Check sheet for the modelled part. Datum: model origin and axes. Units: mm. Face numbers are marked on the shaded views. A direction names the side the tool comes from. Round coordinates to 2 decimals unless told otherwise and drop trailing zeros. Write each loop counter-clockwise with the first axis right and the second up, starting at its lowest first coordinate (ties: lowest second). Pieces come first, ordered by that corner, then holes.
Item 1: Cross-section at A-A on y = 5. Enter the section's corners in (x, z), plus the area to 3 significant figures.
Item 2: Material ranges on line 1 (Y direction, x = -2.5, z = 0); line 2 (X direction, y = 0.75, z = 0); line 3 (X direction, y = 6.25, z = 4.75), recorded low to high.
Item 3: Tool access check on the marked faces 1, 2 and 3. Record the directions out of +Z, -Z, +X, -X, +Y, -Y that give a thin tool (end or side, any length) a straight path to the whole face; none if there is none.
Item 4: Release check for a two-part mould opening along X. For the marked faces 4, 5, 6 and 7 record: +X half, -X half, draft (parallel to the pull), parting line (faces both ways), or undercut.
Item 5: Cross-section at B-B on z = 0. Enter the section's corners in (x, y), plus the area to 3 significant figures.
Item 6: Cross-section at D-D on x = -8.5. Enter the section's corners in (y, z), plus the area to 3 significant figures.
Item 7: Cross-section at C-C on x = -2.75. Enter the section's corners in (y, z), plus the area to 3 significant figures.
Item 8: Go/stop test with flat-tipped pins: pin 1 Ø1 at (x, y) = (-7, 5) entering from -Z; pin 2 Ø3 at (x, z) = (-3, 4.5) entering from -Y. Record where each tip stops, or that it passes through.
from build123d import *

# Parameters (mm, degrees)
SKETCH2_W               = 8
SKETCH2_H               = 10
BOSS_EXTRUDE1_DEPTH     = 8
SKETCH4_W               = 19
SKETCH4_H               = 10
BOSS_EXTRUDE2_DEPTH     = 2
SKETCH6_W               = 19
SKETCH6_H               = 4
BOSS_EXTRUDE3_DEPTH     = 1
SKETCH7_W               = 1
SKETCH7_H               = 10
BOSS_EXTRUDE4_DEPTH     = 2
CUT_EXTRUDE1_REACH      = 24.293
SKETCH3_R               = 2.5
CUT_EXTRUDE2_REACH      = 21
CUT_EXTRUDE2_END_RADIUS = 2.5
SKETCH8_R               = 1
FILLET3_R               = 4
SKETCH9_W               = 10
SKETCH9_H               = 10
CUT_EXTRUDE3_DEPTH      = 0.5


with BuildPart() as part:
    # Sketch2 → Boss-Extrude1 (new body)
    with BuildSketch(Plane(origin=(0, 0, 0), x_dir=(1, 0, 0), z_dir=(0, 1, 0))):
        Rectangle(SKETCH2_W, SKETCH2_H)
    extrude(amount=BOSS_EXTRUDE1_DEPTH)

    # Sketch4 → Boss-Extrude2 (add)
    with BuildSketch(Plane(origin=(0, 8, 0), x_dir=(1, 0, 0), z_dir=(0, 1, 0))):
        with Locations((-5.5, 0)):
            Rectangle(SKETCH4_W, SKETCH4_H)
    extrude(amount=BOSS_EXTRUDE2_DEPTH)

    # Sketch6 → Boss-Extrude3 (add)
    with BuildSketch(Plane.XY.offset(5)):
        with Locations((-5.5, 8)):
            Rectangle(SKETCH6_W, SKETCH6_H)
    boss_extrude3 = extrude(amount=BOSS_EXTRUDE3_DEPTH)

    # Mirror1: Boss-Extrude3 across plane
    add(boss_extrude3.mirror(Plane.XY))

    # Sketch7 → Boss-Extrude4 (add)
    with BuildSketch(Plane.XZ.offset(-8)):
        with Locations((-14.5, 0)):
            Rectangle(SKETCH7_W, SKETCH7_H)
    extrude(amount=BOSS_EXTRUDE4_DEPTH)

    # Sketch3 → Cut-Extrude1 (cut, up to next)
    with BuildSketch(Plane(origin=(4, 0, 0), x_dir=(0, 0, -1), z_dir=(1, 0, 0)), mode=Mode.PRIVATE) as cut_extrude1_sk1:
        with Locations((0, 5)):
            Circle(SKETCH3_R)
    cut_extrude1_tool1 = extrude(cut_extrude1_sk1.sketch, amount=-CUT_EXTRUDE1_REACH, mode=Mode.PRIVATE) & part.part
    add(cut_extrude1_tool1.solids().sort_by_distance((4, 5, 0))[0], mode=Mode.SUBTRACT)

    # Cut-Extrude2: up to this cylinder (the profile starts outside it)
    cut_extrude2_end = Plane(origin=(0, 5, 0), z_dir=(1, 0, 0)) * Cylinder(CUT_EXTRUDE2_END_RADIUS, 48, mode=Mode.PRIVATE)
    # Sketch8 → Cut-Extrude2 (cut, up to the surface)
    with BuildSketch(Plane.XZ, mode=Mode.PRIVATE) as cut_extrude2_sk1:
        with Locations(Location((0, 0, 0), (0, 0, 270))):
            Circle(SKETCH8_R)
    cut_extrude2_tool1 = extrude(cut_extrude2_sk1.sketch, amount=-CUT_EXTRUDE2_REACH, mode=Mode.PRIVATE) - cut_extrude2_end
    add(cut_extrude2_tool1.solids().sort_by_distance((0, 0, 0))[0], mode=Mode.SUBTRACT)

    # Fillet3
    fillet3_edges = [part.edges().sort_by_distance(p)[0] for p in [
        (0, 0, 5),
        (0, 0, -5),
    ]]
    fillet(fillet3_edges, radius=FILLET3_R - 0.0001)  # a hair under: the kernel refuses the full size

    # Sketch9 → Cut-Extrude3 (cut)
    with BuildSketch(Plane(origin=(0, 10, 0), x_dir=(1, 0, 0), z_dir=(0, 1, 0))):
        with Locations((-9, 0)):
            Rectangle(SKETCH9_W, SKETCH9_H)
    extrude(amount=-CUT_EXTRUDE3_DEPTH, mode=Mode.SUBTRACT)


solid = part.part
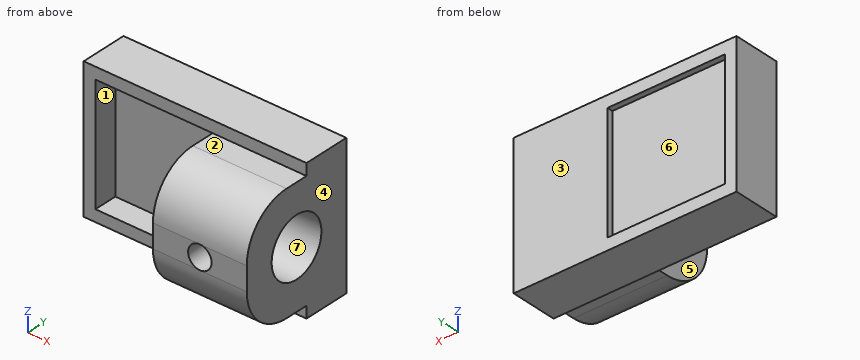
Response values:
1. outline: (-4, -5) - (4, -5) - (4, -2.5) - (-4, -2.5) - close; (-4, 2.5) - (4, 2.5) - (4, 5) - (-4, 5) - close
1. area: 40.0 mm2
2. line 1: y = 0 to 2.5, 7.5 to 10
2. line 2: x = -4 to -1, 1 to 4
2. line 3: x = -15 to -14, -4 to 4
3. face 1: -Y
3. face 2: +Z, +X, -X, -Y
3. face 3: +Z, -Z, +X, -X, +Y
4. face 4: +X half
4. face 5: undercut
4. face 6: undercut
4. face 7: draft
5. outline: (-15, 6) - (-14, 6) - (-14, 8) - (-4, 8) - (-4, 7.5) - (4, 7.5) - (4, 10) - (-4, 10) - (-4, 9.5) - (-14, 9.5) - (-14, 10) - (-15, 10) - close; (-4, 0) - (-1, 0) - (-1, 2.5) - (-4, 2.5) - close; (1, 0) - (4, 0) - (4, 2.5) - (1, 2.5) - close
5. area: 54.0 mm2
6. outline: (6, -6) - (10, -6) - (10, -5) - (9.5, -5) - (9.5, 5) - (10, 5) - (10, 6) - (6, 6) - (6, 5) - (8, 5) - (8, -5) - (6, -5) - close
6. area: 23.0 mm2
7. outline: (0, -1) arc R4 ccw to (4, -5) - (6, -5) - (6, -6) - (10, -6) - (10, 6) - (6, 6) - (6, 5) - (4, 5) arc R4 ccw to (0, 1) - close; hole circle Ø5 at (5, 0)
7. area: 81.5 mm2
8. pin 1: passes through
8. pin 2: stops at y = 0.54
